Can you work these out from the model? Positions are in its coordinate system, mm. A direction names the side the tool comes from. Coordinates: 2 decimals unless noted, no trailing zeros. Write each loop counter-clockwise with the first axis right and the second up, starting at its lowest first coordinate (ties: lowest second). Pieces come first, ordered by that corner, then holes. Notation, with made-up numbers: (-9, -3.5) - (5, -3.5) arc R24 ccw to (5, 24.5) - close; hole circle Ø11 at (-15, 0.25). An arc over 180 degrees is marked (long way). Use one line per item in the form item = value. Start each with the question number.
(1) Thinking about a two-plate mould opening in X: for faces 1 (the face through (-74.5, -13.1, -1.3)), 2 (the face through (-56.5, 0, 7)), 3 (the face through (-80.42, 15.62, -3.47)), 4 (the face through (-71.5, 13.4, 0.3)), which applies, pulls with the +X half, pulls with the -X half, needs draft (parallel to the pull), parting line crosses it, or undercut?
(2) On a 3-axis mill with a long thin cutter (end or side, diameter ignored), from which of +Z, -Z, +X, -X, +Y, -Y can I reach the whole of each face in a straight line? I mean faces 5 (the face through (-87.24, -7.509, 23.846)), 6 (the face through (-64.5, 11, 12)), 7 (the face through (-20, 20.2, 0.4)). Say none if no direction works.
(3) If we section it at B-B on x = -11: Please give me the cut outline in (y, z).
(4) For pin 1 Ø1.5 at (x, z) = (-37.5, 3) entering from +Y; pin 2 Ø8 at (x, y) = (-53, -16) entering from -Z; pin 3 Ø15.5 at (y, z) = (0, 0) entering from -X, each with a flat end and sliding along its axis, tell me the tip position at first contact or that it passes through.
(5) If I drill on probe 1 along Z at (x, y) = (-73, 0); probe 2 along X at (y, z) = (2, -14); probe 3 along Z at (x, y) = (-66, 0), over which ranges is the centre line in solid material (lowest first)? Write a range as from..to.
(6) If we section it at A-A on x = -70: Please give me the cut outline in (y, z), then the cut area to 3 significant figures.
```python
from build123d import *


with BuildPart() as f1:
    # F0 (on Front) → F1 (revolve)
    with BuildSketch(Plane.XZ):
        with BuildLine():
            Line((-56.5, 6), (0, 6))
            Line((0, 6), (0, 16))
            Line((0, 16), (-3, 16))
            Line((-3, 16), (-3, 20))
            Line((-3, 20), (-20, 20))
            Line((-20, 20), (-20, 31))
            Line((-20, 31), (-32, 31))
            ThreePointArc((-32, 31), (-38, 25), (-44, 31))
            Line((-44, 31), (-82, 31))
            ThreePointArc((-82, 31), (-86.242641, 29.242641), (-88, 25))
            Line((-88, 25), (-86.5, 25))
            Line((-86.5, 25), (-86.5, 16))
            Line((-86.5, 16), (-74.5, 16))
            Line((-74.5, 16), (-74.5, 13))
            Line((-74.5, 13), (-71.5, 13))
            Line((-71.5, 13), (-71.5, 20.5))
            Line((-71.5, 20.5), (-64.5, 20.5))
            Line((-64.5, 20.5), (-64.5, 16))
            Line((-64.5, 16), (-56.5, 16))
            Line((-56.5, 16), (-56.5, 6))
        make_face()
    revolve(axis=Axis((-44, 0, 0), (1, 0, 0)))


solid = f1.part
```
Reported:
q1.face_1 = pulls with the -X half
q1.face_2 = undercut
q1.face_3 = needs draft
q1.face_4 = undercut
q2.face_5 = -X
q2.face_6 = none
q2.face_7 = +X
q3.outline = circle Ø40 at (0, 0); hole circle Ø12 at (0, 0)
q4.pin_1 = 24.97
q4.pin_2 = -28.58
q4.pin_3 = -56.5
q5.probe_1 = -31..-13, 13..31
q5.probe_2 = -74.5..-71.5, -56.5..0
q5.probe_3 = -31..-20.5, 20.5..31
q6.outline = circle Ø62 at (0, 0); hole circle Ø41 at (0, 0)
q6.area = 1,700 mm2
